Design review of the part built by this model. Coordinates are the model's own, in mm. Face numbers are marked on the shaded views. A direction names the side the tool comes from. Coordinates: 2 decimals unless noted, no trailing zeros. Loops run counter-clockwise (first coordinate to the right, second up) from the corner with the lowest first, then second, coordinate; pieces in that order, holes last. Notation, with made-up numbers: M 65.25,46 L 72.25,46 A8 ccw 72.25,60 Z; hole C 50.25,54.25 d7. An arc over 180 degrees is marked long. One line per item, written item: value.
```python
from build123d import *

# Parameters (mm, degrees)
SKETCH1_W           = 74.8
SKETCH1_H           = 74.8
BOSS_EXTRUDE1_DEPTH = 2.3375
SKETCH2_W           = 56.1
SKETCH2_H           = 56.1
BOSS_EXTRUDE2_DEPTH = 7.5
CHAMFER1_SIZE       = 0.25
CUT_EXTRUDE1_DEPTH  = 6.233333333
SKETCH4_R           = 1
CUT_EXTRUDE2_DEPTH  = 4


with BuildPart() as part:
    # Sketch1 → Boss-Extrude1 (new body)
    with BuildSketch(Plane(origin=(0, 0, 0), x_dir=(1, 0, 0), z_dir=(0, 1, 0))):
        with Locations((37.4, 37.4)):
            Rectangle(SKETCH1_W, SKETCH1_H)
    extrude(amount=BOSS_EXTRUDE1_DEPTH)

    # Sketch2 → Boss-Extrude2 (add)
    with BuildSketch(Plane(origin=(0, 0, 0), x_dir=(1, 0, 0), z_dir=(0, 1, 0))):
        with Locations((37.4, 37.4)):
            Rectangle(SKETCH2_W, SKETCH2_H)
    extrude(amount=-BOSS_EXTRUDE2_DEPTH)

    # Chamfer1
    chamfer1_edges = [part.edges().sort_by_distance(p)[0] for p in [
        (9.35, -7.5, -37.4),
        (37.4, -7.5, -65.45),
        (65.45, -7.5, -37.4),
        (37.4, -7.5, -9.35),
        (9.35, 0, -37.4),
        (37.4, 0, -9.35),
        (65.45, 0, -37.4),
        (37.4, 0, -65.45),
    ]]
    chamfer(chamfer1_edges, length=CHAMFER1_SIZE)

    # Sketch3 → Cut-Extrude1 (cut)
    with BuildSketch(Plane(origin=(0, 2.3375, 0), x_dir=(1, 0, 0), z_dir=(0, 1, 0))):
        with BuildLine():
            Line((61.1125, 63.1125), (13.6875, 63.1125))
            ThreePointArc((13.6875, 63.1125), (12.273286438, 62.526713562), (11.6875, 61.1125))
            Line((11.6875, 61.1125), (11.6875, 13.6875))
            ThreePointArc((11.6875, 13.6875), (12.273286438, 12.273286438), (13.6875, 11.6875))
            Line((13.6875, 11.6875), (61.1125, 11.6875))
            ThreePointArc((61.1125, 11.6875), (62.526713562, 12.273286438), (63.1125, 13.6875))
            Line((63.1125, 13.6875), (63.1125, 61.1125))
            ThreePointArc((63.1125, 61.1125), (62.526713562, 62.526713562), (61.1125, 63.1125))
        make_face()
    extrude(amount=-CUT_EXTRUDE1_DEPTH, mode=Mode.SUBTRACT)

    # Sketch4 → Cut-Extrude2 (cut)
    with BuildSketch(Plane(origin=(0, -3.895833333, 0), x_dir=(1, 0, 0), z_dir=(0, 1, 0))):
        with Locations(Location((13.1125, 37.4075, 0), (0, 0, 270))):
            Circle(SKETCH4_R)
        with Locations(Location((21.808611106, 37.4075, 0), (0, 0, 270))):
            Circle(SKETCH4_R)
        with Locations(Location((32.198611106, 37.4075, 0), (0, 0, 270))):
            Circle(SKETCH4_R)
        with Locations(Location((42.588611106, 37.4075, 0), (0, 0, 270))):
            Circle(SKETCH4_R)
        with Locations(Location((52.982499988, 37.4025, 0), (0, 0, 270))):
            Circle(SKETCH4_R)
        with Locations(Location((61.6825, 37.4075, 0), (0, 0, 270))):
            Circle(SKETCH4_R)
    extrude(amount=-CUT_EXTRUDE2_DEPTH, mode=Mode.SUBTRACT)


solid = part.part
```
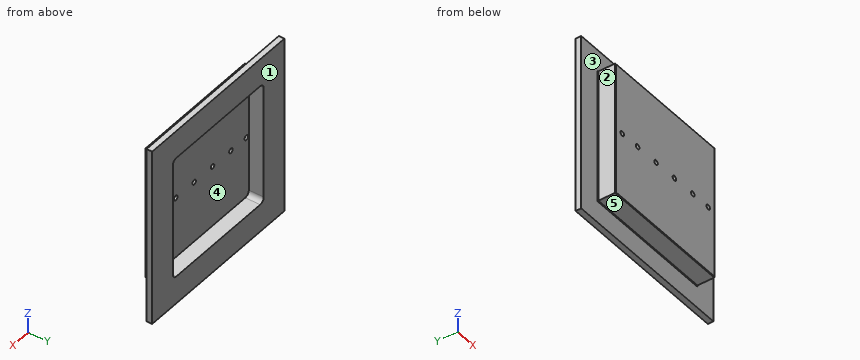
(1) We need section A-A on y = -1.5. State the section outline as (x, z) points, then the cut area to 3 significant figures.
Reply:
outline: M 9.35,-65.45 L 65.45,-65.45 L 65.45,-9.35 L 9.35,-9.35 Z; hole M 11.69,-61.11 A2 ccw 13.69,-63.11 L 61.11,-63.11 A2 ccw 63.11,-61.11 L 63.11,-13.69 A2 ccw 61.11,-11.69 L 13.69,-11.69 A2 ccw 11.69,-13.69 Z
area: 506 mm2
(2) Tool access review of the marked faces 1 and 2: name each direction out of +Z, -Z, +X, -X, +Y, -Y from which nothing blocks a thin tool from reaching the whole face with its end or side.
Reply:
face 1: +Z, -Z, +X, -X, +Y
face 2: +Z, -Z, -X, -Y
(3) We need section D-D on y = -6. State the section outline as (x, z) points, then the cut area to 3 significant figures.
Reply:
outline: M 9.35,-65.45 L 65.45,-65.45 L 65.45,-9.35 L 9.35,-9.35 Z; hole C 13.11,-37.41 d2; hole C 21.81,-37.41 d2; hole C 32.2,-37.41 d2; hole C 42.59,-37.41 d2; hole C 52.98,-37.4 d2; hole C 61.68,-37.41 d2
area: 3,130 mm2
(4) Mouldability with a two-part tool opening along Z and no side actions: class the marked faces 3, 4 and 5 as released by +Z, released by -Z, zero draft, split by the parting line, or undercut.
Reply:
face 3: zero draft
face 4: undercut
face 5: released by -Z
(5) To check wall thickness, follow line 1 along X through (y, z) = (1.25, -45); line 2 along Z through (x, y) = (43, -0.5); line 3 along Z through (x, y) = (15, 1). State the ranges of each line that lie inside material, in increasing order. Write a range as [from, to].
Reply:
line 1: x = [0, 11.69], [63.11, 74.8]
line 2: z = [-65.45, -63.11], [-11.69, -9.35]
line 3: z = [-74.8, -63.11], [-11.69, 0]
(6) Insertion check: pin 1 (2 mm diameter, centred on x = 26.5, y = -4.5, fed in from +Z); pin 2 (3.5 mm diameter, centred on y = -4, z = -39.5, fed in from +X); pin 3 (1 mm diameter, centred on x = 38.5, z = -56, fed in from +Y). Each pin has a flat end and moves straight along its axis. Give the tip position at first contact, or say it passes through.
Reply:
pin 1: stops at z = -9.35
pin 2: stops at x = 65.45
pin 3: stops at y = -3.9
(7) We need section B-B on x = 35.5. State the section outline as (y, z) points.
Reply:
outline: M -7.5,-65.2 L -7.25,-65.45 L -0.25,-65.45 L 0,-65.7 L 0,-74.8 L 2.34,-74.8 L 2.34,-63.11 L -3.9,-63.11 L -3.9,-11.69 L 2.34,-11.69 L 2.34,0 L 0,0 L 0,-9.1 L -0.25,-9.35 L -7.25,-9.35 L -7.5,-9.6 Z
(8) We need section C-C on z = -23.5. State the section outline as (x, y) points.
Reply:
outline: M 0,0 L 9.1,0 L 9.35,-0.25 L 9.35,-7.25 L 9.6,-7.5 L 65.2,-7.5 L 65.45,-7.25 L 65.45,-0.25 L 65.7,0 L 74.8,0 L 74.8,2.34 L 63.11,2.34 L 63.11,-3.9 L 11.69,-3.9 L 11.69,2.34 L 0,2.34 Z
